from build123d import *

# Parameters (mm, degrees)
F0_W     = 76.2
F0_H     = 25.4
F1_DEPTH = 158.75
F2_R     = 12.7
F3_DEPTH = 25.4


with BuildPart() as f1:
    # F0 (on Top) → F1 (new body)
    with BuildSketch(Plane.XY):
        with Locations((1.475252, 0)):
            Rectangle(F0_W, F0_H)
    extrude(amount=F1_DEPTH)

    # F2 (on face) → F3 (cut)
    with BuildSketch(Plane.XZ.offset(12.7)):
        with Locations((0, 111.450641)):
            Circle(F2_R)
        with Locations((0, 47.299359)):
            Circle(F2_R)
    extrude(amount=-F3_DEPTH, mode=Mode.SUBTRACT)


solid = f1.part
Input: part model. Units: mm. Frame: model coordinates. Coordinates: 2 decimals unless noted, no trailing zeros. Loops run counter-clockwise (first coordinate to the right, second up) from the corner with the lowest first, then second, coordinate; pieces in that order, holes last.
Q1. Cut plane C-C (y = -8.25). Output: boundary loops of the cut face in (x, z), then the cut area to 3 significant figures.
Q2. Cut plane A-A (x = 0). Output: boundary loops of the cut face in (y, z), then the cut area to 3 significant figures.
Q3. Material intervals for line 1 (Z direction, x = 0, y = 2); line 2 (Z direction, x = 3, y = -7.75); line 3 (X direction, y = -11.25, z = 41), sorted ascending.
Q4. Cut plane B-B (z = 101). Output: boundary loops of the cut face in (x, y).
Q5. Draft query along X for faces 1 (the face through (1, 12.7, 78)), 2 (the face through (-36.625, 0, 78)), 3 (the face through (-2.75, -0.18, 99.05)). Return one class per face: +X half, -X half, draft (parallel to the pull), parting line (faces both ways), or undercut.
Working result:
1. outline: (-36.62, 0) - (39.58, 0) - (39.58, 158.75) - (-36.62, 158.75) - close; hole circle Ø25.4 at (0, 47.3); hole circle Ø25.4 at (0, 111.45)
1. area: 11,100 mm2
2. outline: (-12.7, 0) - (12.7, 0) - (12.7, 34.6) - (-12.7, 34.6) - close; (-12.7, 60) - (12.7, 60) - (12.7, 98.75) - (-12.7, 98.75) - close; (-12.7, 124.15) - (12.7, 124.15) - (12.7, 158.75) - (-12.7, 158.75) - close
2. area: 2,740 mm2
3. line 1: z = 0 to 34.6, 60 to 98.75, 124.15 to 158.75
3. line 2: z = 0 to 34.96, 59.64 to 99.11, 123.79 to 158.75
3. line 3: x = -36.62 to -11.03, 11.03 to 39.58
4. outline: (-36.62, -12.7) - (-7.22, -12.7) - (-7.22, 12.7) - (-36.62, 12.7) - close; (7.22, -12.7) - (39.58, -12.7) - (39.58, 12.7) - (7.22, 12.7) - close
5. face 1: draft
5. face 2: -X half
5. face 3: undercut
